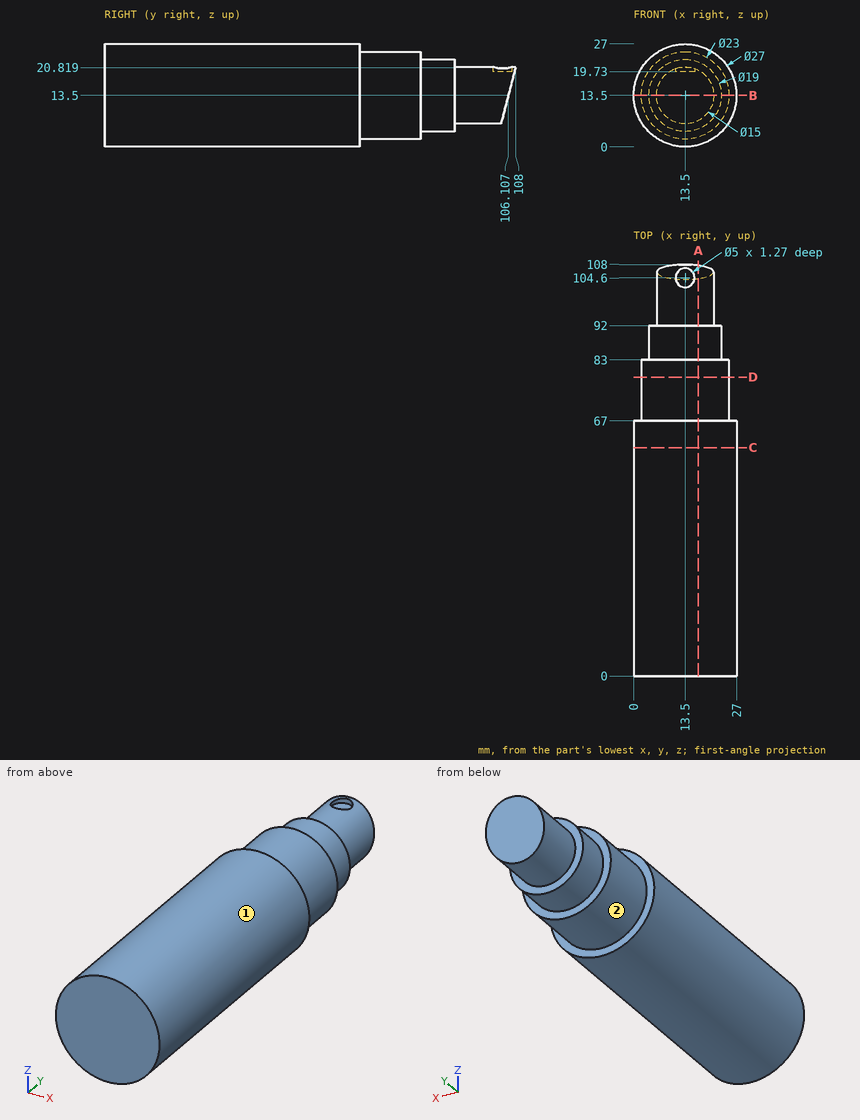
Geometry: see drawing. Coordinates: mm, zero at the bounding-box minimum. A direction names the side the tool comes from. Coordinates: 2 decimals unless noted, no trailing zeros. Order: outer loops, then holes, each group sorted by start corner. A loop starts at its lowest first (then second) coordinate and runs counter-clockwise, first axis right, second up. Notation, with made-up numbers: (87, 66.25) - (91, 66.25) arc R33 ccw to (91, 102.25) - close; hole circle Ø11 at (-34.5, 57). An arc over 180 degrees is marked (long way). Write each question's results on one line, items separated by ' | '.
(1) Set-up query: the marked faces 1 and 2. Return all of +Z, -Z, +X, -X, +Y, -Y with unobstructed straight access to the full face (end or side cutting, diameter ignored); none if empty.
Values found:
face 1: +Y, -Y | face 2: +Y
(2) First-contact query: pin 1 Ø7 at (x, z) = (13.5, 12) entering from +Y (1 decimal); pin 2 Ø6.5 at (x, y) = (13.5, 104.6) entering from +Z; pin 3 Ø1.5 at (y, z) = (34, 18.5) entering from +X. Flat tips, straight axial feed; report the tip coordinate or a pass-through.
Values found:
pin 1: stops at y = 106.6 | pin 2: stops at z = 21 | pin 3: stops at x = 26.31
(3) Section query C-C, the plane y = 60. Return the cut outline in (x, z).
Values found:
outline: circle Ø27 at (13.5, 13.5)
(4) Section query D-D, the plane y = 78.5. Return the cut outline in (x, z).
Values found:
outline: circle Ø23 at (13.5, 13.5)
(5) Line query: line 1 (Y direction, x = 11, z = 21.5); line 2 (Y direction, x = 13.5, z = 20); line 3 (Y direction, x = 13.5, z = 20.4). Output: solid intervals per line, ascending. Write a range as [from, to].
Values found:
line 1: y = [0, 92] | line 2: y = [0, 102.1], [107.1, 107.79] | line 3: y = [0, 102.1], [107.1, 107.89]
(6) Section query A-A, the plane x = 17. Return the cut outline in (y, z) (1 decimal), plus the area to 3 significant figures.
Values found:
outline: (0, 0.5) - (67, 0.5) - (67, 2.5) - (83, 2.5) - (83, 4.7) - (92, 4.7) - (92, 6.9) - (104.4, 6.9) - (107.8, 20.1) - (92, 20.1) - (92, 22.3) - (83, 22.3) - (83, 24.5) - (67, 24.5) - (67, 26.5) - (0, 26.5) - close | area: 2,440 mm²
(7) Section query B-B, the plane z = 13.5. Return the cut outline in (x, y).
Values found:
outline: (0, 0) - (27, 0) - (27, 67) - (25, 67) - (25, 83) - (23, 83) - (23, 92) - (21, 92) - (21, 106.11) - (6, 106.11) - (6, 92) - (4, 92) - (4, 83) - (2, 83) - (2, 67) - (0, 67) - close
